Input: part model. Units: mm. Frame: model coordinates. Coordinates: 2 decimals unless noted, no trailing zeros. Loops run counter-clockwise (first coordinate to the right, second up) from the corner with the lowest first, then second, coordinate; pieces in that order, holes last.
Item 1: Section D-D on y = -1.5. Return loops of the section in (x, z) (1 decimal).
Item 2: Section C-C on y = -22. Return loops of the section in (x, z) (1 decimal).
Item 3: Ray query, line 1 along Z through (x, y) = (0, -10); line 2 along Z through (x, y) = (15, -8). Return the intervals inside material, ascending.
Item 4: Contact query for flat-ended pins moving along their axis: P1, Ø5, axis at x = -19.5, y = 3.5, coming from the +Z side; P2, Ø10, axis at y = 10.5, z = -19.5, coming from the +X side; P3, Ø4, axis at x = -1, y = 8, coming from the -Z side; P4, Ø5, axis at x = -0.5, z = -16, coming from the -Y side. Output: stop coordinate, or through.
Item 5: Pull-direction query (Y, two-part tool) for faces 1 (the flat face through (-17, -25.4, -5)), 2 (the cylindrical face through (18.897, 0.006, -14.49)), 3 (the cylindrical face through (-5.506, -13.731, -24.796)); classes: released by +Y, released by -Y, zero draft, split by the parting line, or undercut.
```python
from build123d import *

# Parameters (mm, degrees)
F0_R      = 25.4
F0_R_2    = 17.4625
F1_DEPTH  = 25.4
F2_R      = 25.4
F2_R_2    = 23.8125
F3_DEPTH  = 3.175
F4_DEPTH  = 3.175
F5_R      = 25.4
F6_DEPTH  = 25.4
F8_SIZE   = 0.8128
F9_R      = 17.4625
F10_DEPTH = 53.976


# Not quite as in the source:
# - a fillet or chamfer that OpenCascade refuses, or shapes differently, is made with other operations: its cross-section is extruded or revolved along the edge and cut away or added


with BuildPart() as f1:
    # F0 (on Front) → F1 (new body)
    with BuildSketch(Plane.XZ):
        Circle(F0_R)
        Circle(F0_R_2, mode=Mode.SUBTRACT)
    extrude(amount=F1_DEPTH)

    # F2 (on face) → F3 (cut)
    with BuildSketch(Plane(origin=(0, 0, 0), x_dir=(-1, 0, 0), z_dir=(0, 1, 0))):
        Circle(F2_R)
        Circle(F2_R_2, mode=Mode.SUBTRACT)
    extrude(amount=-F3_DEPTH, mode=Mode.SUBTRACT)

    # F4 (add): a face of the model
    f4_faces = [f1.faces().sort_by_distance(p)[0] for p in [
        (23.1389807909, 0, 0),
    ]]
    extrude(f4_faces, amount=F4_DEPTH)

    # F5 (on face) → F6 (join)
    with BuildSketch(Plane(origin=(0, 3.175, 0), x_dir=(-1, 0, 0), z_dir=(0, 1, 0))):
        Circle(F5_R)
    extrude(amount=F6_DEPTH)

    # F7: fillet of radius 3.175 on 2 edges, made by hand

    # F7_s1 → F7_t2 (revolve)
    with BuildSketch(Plane.XY):
        with BuildLine():
            ThreePointArc((-23.8125, -0.425369343), (-24.237869343, -2.012869343), (-25.4, -3.175))
            Line((-25.4, -3.175), (-23.8125, -3.175))
            Line((-23.8125, -3.175), (-23.8125, -0.425369343))
        make_face()
    revolve(axis=Axis((0, -3.175, 0), (0, 1, 0)))

    # F7_s3 → F7_t4 (revolve)
    with BuildSketch(Plane.XY):
        with BuildLine():
            ThreePointArc((-25.4, 3.175), (-24.237869343, 2.012869343), (-23.8125, 0.425369343))
            Line((-23.8125, 0.425369343), (-23.8125, 3.175))
            Line((-23.8125, 3.175), (-25.4, 3.175))
        make_face()
    revolve(axis=Axis((0, 3.175, 0), (0, 1, 0)))

    # F8
    f8_edges = [f1.edges().sort_by_distance(p)[0] for p in [
        (-25.4, -25.4, 0),
        (25.4, 28.575, 0),
    ]]
    chamfer(f8_edges, length=F8_SIZE)

    # F9 (on face) → F10 (cut, through all)
    with BuildSketch(Plane(origin=(0, 28.575, 0), x_dir=(-1, 0, 0), z_dir=(0, 1, 0))):
        Circle(F9_R)
    extrude(amount=-F10_DEPTH, mode=Mode.SUBTRACT)


solid = f1.part
```
Results found:
1. outline: circle Ø48 at (0, 0); hole circle Ø34.9 at (0, 0)
2. outline: circle Ø50.8 at (0, 0); hole circle Ø34.9 at (0, 0)
3. line 1: z = -25.4 to -17.46, 17.46 to 25.4
3. line 2: z = -20.5 to -8.94, 8.94 to 20.5
4. P1: stops at z = 18.87
4. P2: stops at x = 20.85
4. P3: stops at z = -25.4
4. P4: stops at y = -25.4
5. face 1: released by -Y
5. face 2: undercut
5. face 3: zero draft
